```python
from build123d import *

# Parameters (mm, degrees)
BODY_DEPTH     = 112
SKETCH2_W      = 71.382300335
SKETCH2_H      = 2.6
TAB_LOW_DEPTH  = 3
SKETCH3_W      = 71.382300335
SKETCH3_H      = 2.6
TAB_HIGH_DEPTH = 3


with BuildPart() as part:
    # Sketch1 → Body (new body)
    with BuildSketch(Plane.XY.offset(3)):
        Polygon((26.524366133, -97.918141453), (99.906666468, -97.918141453), (114.906666468, -96.668141453), (114.906666468, -96.168141453), (99.906666468, -94.918141453), (26.524366133, -94.918141453), align=None)
    extrude(amount=BODY_DEPTH)

    # Sketch2 → Tab_low (add)
    with BuildSketch(Plane.XY):
        with Locations((63.215516301, -96.418141453)):
            Rectangle(SKETCH2_W, SKETCH2_H)
    extrude(amount=TAB_LOW_DEPTH)

    # Sketch3 → Tab_high (add)
    with BuildSketch(Plane.XY.offset(115)):
        with Locations((63.215516301, -96.418141453)):
            Rectangle(SKETCH3_W, SKETCH3_H)
    extrude(amount=TAB_HIGH_DEPTH)


solid = part.part
```
Source: CAD feature listing. Evaluate the final solid. Frame: model axes, mm. A direction names the side the tool comes from. Round coordinates to 2 decimals unless told otherwise and drop trailing zeros. Loops run counter-clockwise (first coordinate to the right, second up) from the corner with the lowest first, then second, coordinate; pieces in that order, holes last. Notation, with made-up numbers: M 49,33 L 94,33 A12 ccw 94,54 Z; hole C 28.5,14.25 d10. An arc over 180 degrees is marked long. Use a Markdown table: item, result. Add a question column.
1. Set-up query: faces 1 (the flat face through (63, -95.118, 116)), 2 (the flat face through (63, -97.718, 1)), 3 (the flat face through (63, -97.718, 116)), 4 (the flat face through (27.524, -96, 1)), 5 (the flat face through (98.907, -96, 116)). Return all of +Z, -Z, +X, -X, +Y, -Y with unobstructed straight access to the full face (end or side cutting, diameter ignored); none if empty.
2. Cut plane B-B, the plane y = -95.65. Output: boundary loops of the cut face in (x, z), and give its area (3 significant figures).
3. Contact query for flat-ended pins moving along their axis: pin 1 (3.5 mm diameter, centred on x = 53.5, z = 2, fed in from -Y); pin 2 (0.8 mm diameter, centred on y = -97, z = 1.5, fed in from -X); pin 3 (1.5 mm diameter, centred on x = 59.5, z = 116.5, fed in from +Y); pin 4 (1.5 mm diameter, centred on x = 66, z = 116.5, fed in from -Y). Output: stop coordinate, or through.
4. Cut plane C-C, the plane x = 102. Output: boundary loops of the cut face in (y, z).
5. Ray query, line 1 along Z through (x, y) = (69, -95); line 2 along Y through (x, z) = (108.5, 21); line 3 along Y through (x, z) = (103.5, 51.5). Return the intervals inside material, ascending. Write a range as [from, to].
6. Cut plane A-A, the plane z = 65. Output: boundary loops of the cut face in (x, y), and give its area (3 significant figures).
Solution:
| question | item | result |
|---|---|---|
| 1 | face 1 | +Z, +X, -X, +Y |
| 1 | face 2 | -Z, +X, -X, -Y |
| 1 | face 3 | +Z, +X, -X, -Y |
| 1 | face 4 | -Z, -X, +Y, -Y |
| 1 | face 5 | +Z, +X, +Y, -Y |
| 2 | outline | M 26.52,3 L 27.52,3 L 27.52,0 L 98.91,0 L 98.91,3 L 108.69,3 L 108.69,115 L 98.91,115 L 98.91,118 L 27.52,118 L 27.52,115 L 26.52,115 Z |
| 2 | area | 9,630 mm2 |
| 3 | pin 1 | stops at y = -97.92 |
| 3 | pin 2 | stops at x = 27.52 |
| 3 | pin 3 | stops at y = -95.12 |
| 3 | pin 4 | stops at y = -97.72 |
| 4 | outline | M -97.74,3 L -95.09,3 L -95.09,115 L -97.74,115 Z |
| 5 | line 1 | z = [3, 115] |
| 5 | line 2 | y = [-97.2, -95.63] |
| 5 | line 3 | y = [-97.62, -95.22] |
| 6 | outline | M 26.52,-97.92 L 99.91,-97.92 L 114.91,-96.67 L 114.91,-96.17 L 99.91,-94.92 L 26.52,-94.92 Z |
| 6 | area | 246 mm2 |
